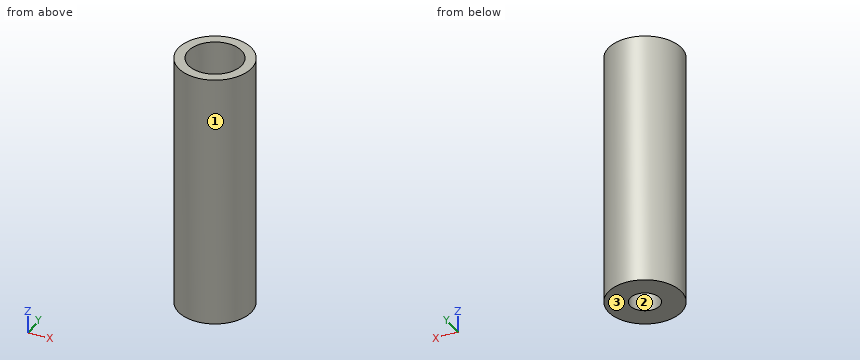
```python
from build123d import *

# Parameters (mm, degrees)
F0_R     = 12.7
F1_DEPTH = 73.66
F2_R     = 5.1125641025
F3_DEPTH = 73.661
F3_TAPER = -2.9356734464
F4_R     = 12.7
F5_DEPTH = 15.24
F8_D     = 18.5
F8_DEPTH = 19.7358
F8_TIP   = 5.557960726


with BuildPart() as f1:
    # F0 (on Top) → F1 (new body)
    with BuildSketch(Plane.XY):
        Circle(F0_R)
    extrude(amount=F1_DEPTH)

    # F2 (on Top) → F3 (cut, through all)
    with BuildSketch(Plane.XY):
        Circle(F2_R)
    extrude(amount=F3_DEPTH, taper=F3_TAPER, mode=Mode.SUBTRACT)

    # F4 (on face) → F5 (join)
    with BuildSketch(Plane.XY.offset(73.66)):
        Circle(F4_R)
    extrude(amount=F5_DEPTH)

    # F8
    with Locations(Plane.XY.offset(88.9)):
        with Locations((0, 0)):
            Hole(F8_D / 2, depth=F8_DEPTH)
            with Locations((0, 0, -(F8_DEPTH + F8_TIP / 2))):  # 118° drill point
                Cone(0, F8_D / 2, F8_TIP, mode=Mode.SUBTRACT)


solid = f1.part
```
Part model, mm, in its own coordinate system. Face numbers are marked on the shaded views. Give positions to 0.01 mm unless a question says otherwise; leave off trailing zeros. Write each loop counter-clockwise with the first axis right and the second up, starting at its lowest first coordinate (ties: lowest second). Pieces come first, ordered by that corner, then holes. Notation, with made-up numbers: (79, -24) -> (88, -24) arc R19 ccw to (88, 2) -> close; hole circle Ø3 at (10, -6.5). An arc over 180 degrees is marked (long way). Put each result on its own line as item: value. Start each with the question number.
Item 1: Cut at B-B (z = 11). List the corners of the cut face in (x, y), then the cut area to 3 significant figures.
Item 2: Pin check, flat tips, straight feed: pin 1 Ø6 at (x, z) = (-6.5, 71.5) entering from +Y; pin 2 Ø3 at (y, z) = (2, 46) entering from -X; pin 3 Ø2 at (x, z) = (9, 21) entering from -Y. Stop position of each tip, or through.
Item 3: Cut at C-C (z = 33). List the corners of the cut face in (x, y), then the cut area to 3 significant figures.
Item 4: Wall check: L1, parallel to Y at x = 0, z = 78.75; L2, parallel to Y at x = -1.75, z = 62.5; L3, parallel to Z at x = -5, y = 7.75. Give the ranges that are in metal, low to high. Write a range as [from, to].
Item 5: Cut at A-A (x = 0). List the corners of the cut face in (y, z), then the cut area to 3 significant figures.
Item 6: Pull direction X, two halves, no side cores. Call the marked faces 1, 2 and 3: pulls with the +X half, pulls with the -X half, needs draft (parallel to the pull), parting line crosses it, or undercut.
Answer list:
1. outline: circle Ø25.4 at (0, 0); hole circle Ø11.35 at (0, 0)
1. area: 405 mm2
2. pin 1: stops at y = 12.21
2. pin 2: stops at x = -12.69
2. pin 3: stops at y = -9.86
3. outline: circle Ø25.4 at (0, 0); hole circle Ø13.61 at (0, 0)
3. area: 361 mm2
4. L1: y = [-12.7, -9.25], [9.25, 12.7]
4. L2: y = [-12.58, -8.13], [8.13, 12.58]
4. L3: z = [0, 69.15]
5. outline: (-12.7, 0) -> (-5.11, 0) -> (-8.64, 68.8) -> (-9.25, 69.16) -> (-9.25, 88.9) -> (-12.7, 88.9) -> close; (5.11, 0) -> (12.7, 0) -> (12.7, 88.9) -> (9.25, 88.9) -> (9.25, 69.16) -> (8.64, 68.8) -> close
5. area: 940 mm2
6. face 1: parting line crosses it
6. face 2: undercut
6. face 3: needs draft
